from build123d import *

# Parameters (mm, degrees)
CUT_EXTRUDE2_DEPTH = 2.31


with BuildPart() as part:
    # Sketch10 → Revolve3 (revolve)
    with BuildSketch(Plane(origin=(0, 0, 0), x_dir=(0, 0, -1), z_dir=(1, 0, 0)), mode=Mode.PRIVATE) as revolve3_sk:
        Polygon((22.55, 3), (23.3, 2.25), (23.3, 0), (3.3, 0), (3.3, 3), align=None)
    revolve(revolve3_sk.sketch.rotate(Axis((0, 0, 0), (0, 0, -1)), 90), axis=Axis((0, 0, 0), (0, 0, -1)))

    # Sketch7 → Revolve2 (revolve)
    with BuildSketch(Plane(origin=(0, 0, 0), x_dir=(0, 0, -1), z_dir=(1, 0, 0)), mode=Mode.PRIVATE) as revolve2_sk:
        with BuildLine():
            Line((2.805, 5.25), (3.3, 5.25))
            Line((3.3, 5.25), (3.3, 0))
            Line((3.3, 0), (0, 0))
            Line((0, 0), (0, 3))
            ThreePointArc((0, 3), (1.216479019, 4.356906156), (2.805, 5.25))
        make_face()
    revolve(revolve2_sk.sketch.rotate(Axis((0, 0, 0), (0, 0, -1)), 180), axis=Axis((0, 0, 0), (0, 0, -1)))

    # Sketch5 → Cut-Extrude2 (cut)
    with BuildSketch(Plane.XY):
        Polygon((2, -1.154700538), (2, 1.154700538), (0, 2.309401077), (-2, 1.154700538), (-2, -1.154700538), (0, -2.309401077), align=None)
    extrude(amount=-CUT_EXTRUDE2_DEPTH, mode=Mode.SUBTRACT)

    # Cut-Extrude3 cone 1 section (through the dimple's axis) → Cut-Extrude3 (revolve, cut)
    with BuildSketch(Plane(origin=(0, 0, 0), x_dir=(0, -1, 0), z_dir=(1, 0, 0))):
        Polygon((0, 0), (2.309401077, 0), (0, 2.309401077), align=None)
    revolve(axis=Axis((0, 0, 0), (0, 0, -1)), mode=Mode.SUBTRACT)


with BuildPart() as body_2:
    # Split1: read off the stored shape, not the designer's step
    # Split1: the piece on the far side of the plane
    add(part.part)
    split(bisect_by=Plane.XY.offset(-3.3), keep=Keep.BOTTOM)


with BuildPart() as part_1:
    add(part.part)

    # Split1
    split(bisect_by=Plane.XY.offset(-3.3), keep=Keep.TOP)


with BuildPart() as body_2_1:
    add(body_2.part)

    # Boss-Extrude1: read off the stored shape, not the designer's step
    # Boss-Extrude1: union part
    add(part_1.part)


solid = body_2_1.part
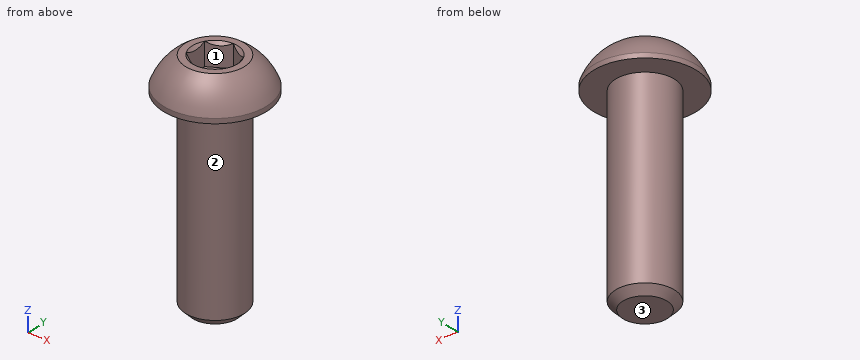
Input: part model. Units: mm. Frame: model coordinates. Face numbers are marked on the shaded views. Give positions to 0.01 mm unless a question says otherwise; leave off trailing zeros. Order: outer loops, then holes, each group sorted by start corner. A loop starts at its lowest first (then second) coordinate and runs counter-clockwise, first axis right, second up. Notation, with made-up numbers: M 57.5,27.5 L 91.5,27.5 A30 cw 91.5,58.5 Z; hole C -28,50.25 d4. An arc over 180 degrees is marked long. Answer as a JSON object with one key per item and string values.
1. Cut plane B-B, the plane z = -6.5. Output: boundary loops of the cut face in (x, y), and give its area (3 significant figures).
Result sheet:
{"outline": "C 0,0 d6", "area": "28.3 mm²"}
2. First-contact query: P1, Ø2, axis at x = -2, z = -7, coming from the -Y side; P2, Ø4, axis at x = 3.5, y = 1.5, coming from the -Z side; P3, Ø5, axis at y = 3.5, z = -19, coming from the -X side; P4, Ø1.2, axis at y = 0, z = -1, coming from the +X side. Flat tips, straight axial feed; report the tip coordinate or a pass-through.
Result sheet:
{"P1": "y = -2.83", "P2": "z = -23.3", "P3": "x = -2.83", "P4": "x = 4.64"}
3. Ray query, line 1 (Z direction, x = -1, y = 1); line 2 (Y direction, x = 0, z = -13.75); line 3 (Y direction, x = 1.75, z = -13). Return the intervals inside material, ascending. Write a range as [from, to].
Result sheet:
{"line 1": "[-23.3, -2.31]", "line 2": "[-3, 3]", "line 3": "[-2.44, 2.44]"}
4. Cut plane C-C, the plane x = -4.5. Output: boundary loops of the cut face in (y, z) (3 decimals), and give its area (3 significant figures).
Result sheet:
{"outline": "M -2.704,-3.3 L 2.704,-3.3 L 2.704,-2.805 A3.309 ccw -2.704,-2.805 Z", "area": "8.00 mm²"}
5. Cut plane A-A, the plane y = 0. Output: boundary loops of the cut face in (x, z) (3 decimals), and give its area (3 significant figures).
Result sheet:
{"outline": "M -5.25,-3.3 L -3,-3.3 L -3,-22.55 L -2.25,-23.3 L 2.25,-23.3 L 3,-22.55 L 3,-3.3 L 5.25,-3.3 L 5.25,-2.805 A5.585 ccw 3,0 L 2.309,0 L 2,-0.309 L 2,-2.31 L -2,-2.31 L -2,-0.309 L -2.309,0 L -3,0 A5.585 ccw -5.25,-2.805 Z", "area": "140 mm²"}
6. Pull-direction query (Y, two-part tool) for the marked faces 1, 2 and 3; classes: +Y half, -Y half, draft (parallel to the pull), parting line (faces both ways), or undercut.
Result sheet:
{"face 1": "undercut", "face 2": "parting line", "face 3": "draft"}
7. Cut plane D-D, the plane y = 4. Output: boundary loops of the cut face in (x, z) (3 decimals), and give its area (3 significant figures).
Result sheet:
{"outline": "M -3.4,-3.3 L 3.4,-3.3 L 3.4,-2.805 A3.898 ccw -3.4,-2.805 Z", "area": "13.0 mm²"}
